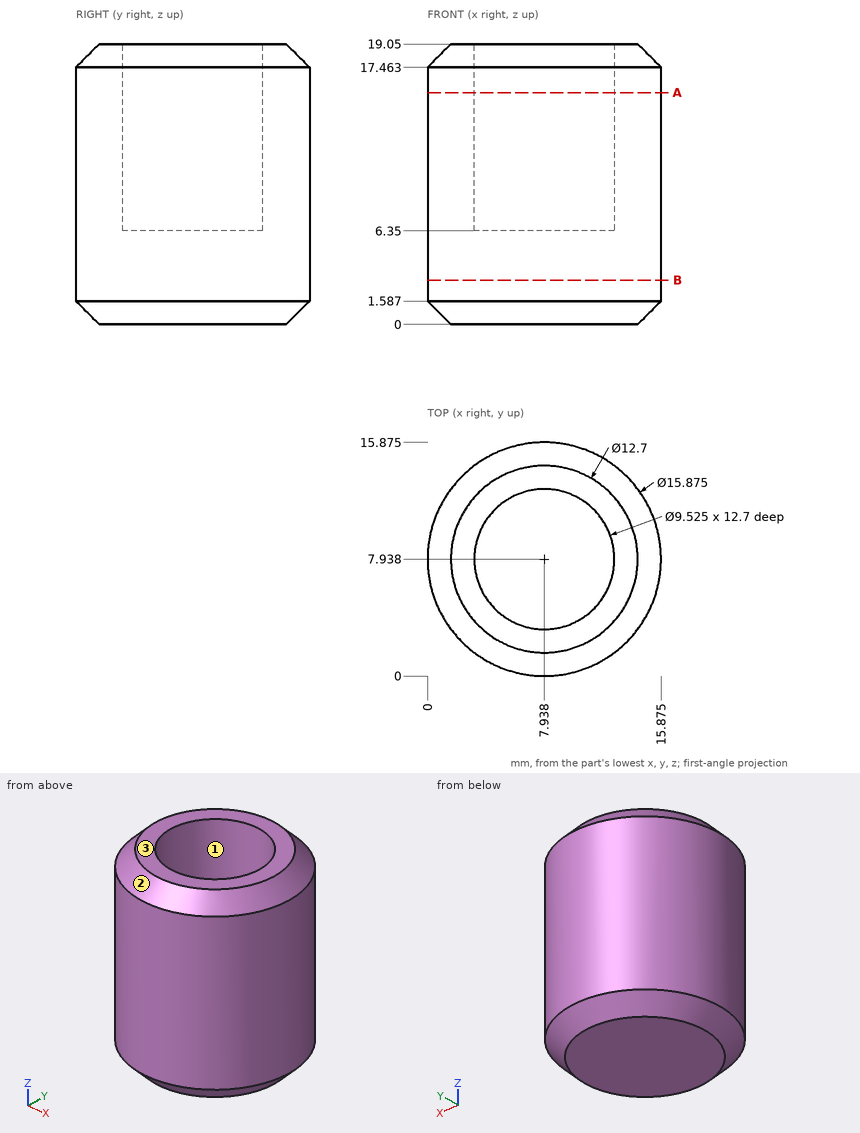
Print and shaded views of the part. All mm, measured from the part's lowest x, y and z. Coordinates: 2 decimals unless noted, no trailing zeros. Loops run counter-clockwise (first coordinate to the right, second up) from the corner with the lowest first, then second, coordinate; pieces in that order, holes last. Notation, with made-up numbers: (-9.75, -8) - (17.25, -8) arc R5 cw to (17.25, -2) - close; hole circle Ø6 at (16.5, -9.5). An arc over 180 degrees is marked (long way). Write item = value, one per line. Start each with the question number.
Item 1: Drop flat-ended pins along their axis: pin 1 Ø5.5 at (x, y) = (7.94, 7.94) entering from -Z; pin 2 Ø2 at (x, z) = (12.5, 6) entering from -Y (1 decimal); pin 3 Ø6 at (x, z) = (13.5, 6.5) entering from +Y; pin 4 Ø3 at (x, y) = (9, 7) entering from +Z. Give the stop position or say it passes through.
Item 2: Wall check: probe 1 along Z at (x, y) = (8.5, 9.75); probe 2 along Y at (x, z) = (8, 7.5) (1 decimal); probe 3 along X at (y, z) = (11.75, 13.75) (1 decimal). Give the ranges that are in metal, low to high. Write a range as [from, to].
Item 3: Pull direction Y, two halves, no side cores. Call the marked faces 1, 2 and 3: +Y half, -Y half, draft (parallel to the pull), parting line (faces both ways), or undercut.
Item 4: Saw through at B-B, the plane z = 3. List the corners of the cut face in (x, y) (1 decimal).
Item 5: Saw through at A-A, the plane z = 15.75. List the corners of the cut face in (x, y) (1 decimal).
Answers:
q1.pin_1 = 0
q1.pin_2 = 0.8
q1.pin_3 = 15.45
q1.pin_4 = 6.35
q2.probe_1 = [0, 6.35]
q2.probe_2 = [0, 3.2], [12.7, 15.9]
q2.probe_3 = [1, 5.1], [10.8, 14.9]
q3.face_1 = undercut
q3.face_2 = parting line
q3.face_3 = draft
q4.outline = circle Ø15.9 at (7.9, 7.9)
q5.outline = circle Ø15.9 at (7.9, 7.9); hole circle Ø9.5 at (7.9, 7.9)
